Geometry check sheet. Reference: the model listing, model coordinates, mm. A direction names the side the tool comes from. Coordinates: 2 decimals unless noted, no trailing zeros. Order: outer loops, then holes, each group sorted by start corner. A loop starts at its lowest first (then second) coordinate and runs counter-clockwise, first axis right, second up. Notation, with made-up numbers: M -6.75,-37 L 40.25,-37 A24 ccw 40.25,-6 Z; hole C 13,41 d4. An arc over 180 degrees is marked long. One line per item, written item: value. Start each with the question number.
1) Sectioned sample at D-D, the plane x = 16. Enter the section's corners in (y, z), then the cut area to 3 significant figures.
2) Go/stop test with flat-tipped pins: P1, Ø2, axis at x = 6, z = -5.5, coming from the -Y side; P2, Ø1.5, axis at x = -11, z = 17.5, coming from the +Y side. Record where each tip stops, or that it passes through.
3) Sectioned sample at B-B, the plane z = 13. Enter the section's corners in (x, y).
4) Sectioned sample at C-C, the plane y = 10.25. Enter the section's corners in (x, z), then the cut area to 3 significant figures.
5) Thickness scan on L1, parallel to Y at x = 16, z = 9; L2, parallel to Z at x = 4, y = 12.5; L3, parallel to Z at x = -8.5, y = 10.5. Record the ranges inside material, lowest first. Write a range as from..to.
6) Sectioned sample at A-A, the plane x = 8. Enter the section's corners in (y, z).
7) Access from +Z, -Z, +X, -X, +Y, -Y to the whole of each face (thin tool, end or side, straight path). Record for faces 1 (the cylindrical face through (2.81, 12.08, -0.07)), 2 (the cylindrical face through (20.58, 4.92, -10.03)).
```python
from build123d import *

# Parameters (mm, degrees)
SKETCH_1_W      = 36.8
SKETCH_1_H      = 36
EXTRUDE_1_DEPTH = 10.7
FILLET_1_R      = 1
SKETCH_2_R      = 7.75
EXTRUDE_2_DEPTH = 2.8


with BuildPart() as part:
    # 草图1 → 凸台-拉伸1 (new body)
    with BuildSketch(Plane(origin=(0, 0, 0), x_dir=(1, 0, 0), z_dir=(0, 1, 0))):
        with Locations((2.46557377, -7.672131148)):
            Rectangle(SKETCH_1_W, SKETCH_1_H)
    extrude(amount=EXTRUDE_1_DEPTH)

    # 圆角1
    fillet_1_edges = [part.edges().sort_by_distance(p)[0] for p in [
        (20.86557377, 10.7, 7.672131148),
        (2.46557377, 10.7, -10.327868852),
        (-15.93442623, 10.7, 7.672131148),
        (-15.93442623, 5.35, -10.327868852),
        (20.86557377, 5.35, -10.327868852),
        (20.86557377, 5.35, 25.672131148),
        (-15.93442623, 5.35, 25.672131148),
        (2.46557377, 10.7, 25.672131148),
    ]]
    fillet(fillet_1_edges, radius=FILLET_1_R)

    # 草图2 → 凸台-拉伸2 (add)
    with BuildSketch(Plane(origin=(0, 10.7, 0), x_dir=(1, 0, 0), z_dir=(0, 1, 0))):
        with Locations(Location((2.46557377, -7.672131148, 0), (0, 0, 270))):
            Circle(SKETCH_2_R)
    extrude(amount=EXTRUDE_2_DEPTH)


solid = part.part
```
Final values:
1. outline: M 0,-10.33 L 9.7,-10.33 A1 ccw 10.7,-9.33 L 10.7,24.67 A1 ccw 9.7,25.67 L 0,25.67 Z
1. area: 385 mm^2
2. P1: stops at y = 0
2. P2: stops at y = 10.7
3. outline: M -15.93,0 L 20.87,0 L 20.87,9.7 A1 ccw 19.87,10.7 L 8.09,10.7 L 8.09,13.5 L -3.16,13.5 L -3.16,10.7 L -14.93,10.7 A1 ccw -15.93,9.7 Z
4. outline: M -15.77,-9.33 A0.84 ccw -14.93,-10.16 L 19.87,-10.16 A0.84 ccw 20.7,-9.33 L 20.7,24.67 A0.84 ccw 19.87,25.51 L -14.93,25.51 A0.84 ccw -15.77,24.67 Z
4. area: 1,300 mm^2
5. L1: y = 0..10.7
5. L2: z = 0.08..15.27
5. L3: z = -9.93..25.27
6. outline: M 0,-10.33 L 9.7,-10.33 A1 ccw 10.7,-9.33 L 10.7,2.25 L 13.5,2.25 L 13.5,13.1 L 10.7,13.1 L 10.7,24.67 A1 ccw 9.7,25.67 L 0,25.67 Z
7. face 1: +Y
7. face 2: -Z, +X, +Y, -Y
